from build123d import *

# Parameters (mm, degrees)
F0_W        = 102
F0_H        = 59.8
F0_W_2      = 98
F0_H_2      = 55.8
F1_DEPTH    = 8
F2_W        = 102.0620055497
F2_H        = 59.6651937813
F3_DEPTH    = 0.6
F4_W        = 100.1025550067
F4_H        = 57.5502440333
F4_W_2      = 98
F4_H_2      = 55.8
F5_DEPTH    = 2.5
F6_T1_DEPTH = 105.5349790349
F6_T3_DEPTH = 3.6684549434
F6_T5_DEPTH = 66.8066222098
F6_T7_DEPTH = 3.6684549117
F6_T9_DEPTH = 105.5349790665
F7_W        = 73
F7_H        = 27
F8_DEPTH    = 8.6010001


# Not quite as in the source:
# - a fillet or chamfer that OpenCascade refuses, or shapes differently, is made with other operations: its cross-section is extruded or revolved along the edge and cut away or added


with BuildPart() as f1:
    # F0 (on Top) → F1 (new body)
    with BuildSketch(Plane.XY):
        with Locations((-11.1629452705, -1.3489569187)):
            Rectangle(F0_W, F0_H)
        with Locations((-11.1629452705, -1.3489569187)):
            Rectangle(F0_W_2, F0_H_2, mode=Mode.SUBTRACT)
    extrude(amount=F1_DEPTH)

    # F2 (on Top) → F3 (join)
    with BuildSketch(Plane.XY):
        with Locations((-11.096207425, -1.3842275366)):
            Rectangle(F2_W, F2_H)
    extrude(amount=-F3_DEPTH)

    # F4 (on face) → F5 (join)
    with BuildSketch(Plane.XY.offset(8)):
        with Locations((-11.0803488642, -1.3563353568)):
            Rectangle(F4_W, F4_H)
        with Locations((-11.1629452705, -1.3489569187)):
            Rectangle(F4_W_2, F4_H_2, mode=Mode.SUBTRACT)
    extrude(amount=F5_DEPTH)

    # F6: fillet of radius 2 on 4 edges, made by hand

    # F6_s2 → F6_t1 (cut)
    with BuildSketch(Plane.YZ.offset(-65.6979244141)):
        with BuildLine():
            ThreePointArc((-29.7885387415, -0.6), (-30.5631354108, -0.4439088915), (-31.2168244272, 0))
            Line((-31.2168244272, 0), (-31.2168244272, -0.6))
            Line((-31.2168244272, -0.6), (-29.7885387415, -0.6))
        make_face()
    extrude(amount=F6_T1_DEPTH, mode=Mode.SUBTRACT)

    # F6_s4 → F6_t3 (cut)
    with BuildSketch(Plane.YZ.offset(39.8370546207)):
        with BuildLine():
            ThreePointArc((-29.7885387415, -0.6), (-30.5631354108, -0.4439088915), (-31.2168244272, 0))
            Line((-31.2168244272, 0), (-31.2168244272, -0.6))
            Line((-31.2168244272, -0.6), (-29.7885387415, -0.6))
        make_face()
    extrude(amount=F6_T3_DEPTH, mode=Mode.SUBTRACT)

    # F6_s6 → F6_t5 (cut)
    with BuildSketch(Plane.XZ.offset(-32.0190835683)):
        with BuildLine():
            ThreePointArc((-60.6989245141, -0.6), (-61.4735211834, -0.4439088915), (-62.1272101998, 0))
            Line((-62.1272101998, 0), (-62.1272101998, -0.6))
            Line((-62.1272101998, -0.6), (-60.6989245141, -0.6))
        make_face()
        with BuildLine():
            ThreePointArc((38.5065096641, -0.6), (39.2811063334, -0.4439088915), (39.9347953498, 0))
            Line((39.9347953498, 0), (39.9347953498, -0.6))
            Line((39.9347953498, -0.6), (38.5065096641, -0.6))
        make_face()
    extrude(amount=F6_T5_DEPTH, mode=Mode.SUBTRACT)

    # F6_s8 → F6_t7 (cut)
    with BuildSketch(Plane.YZ.offset(39.8370546524)):
        with BuildLine():
            ThreePointArc((28.448369354, 0), (27.7946803375, -0.4439088915), (27.0200836683, -0.6))
            Line((27.0200836683, -0.6), (28.448369354, -0.6))
            Line((28.448369354, -0.6), (28.448369354, 0))
        make_face()
    extrude(amount=F6_T7_DEPTH, mode=Mode.SUBTRACT)

    # F6_s10 → F6_t9 (cut)
    with BuildSketch(Plane.YZ.offset(-65.6979244141)):
        with BuildLine():
            ThreePointArc((28.448369354, 0), (27.7946803375, -0.4439088915), (27.0200836683, -0.6))
            Line((27.0200836683, -0.6), (28.448369354, -0.6))
            Line((28.448369354, -0.6), (28.448369354, 0))
        make_face()
    extrude(amount=F6_T9_DEPTH, mode=Mode.SUBTRACT)

    # F7 (on face) → F8 (cut, through all)
    with BuildSketch(Plane.XY.offset(8)):
        with Locations((-6.6629452705, 6.0510430813)):
            Rectangle(F7_W, F7_H)
    extrude(amount=-F8_DEPTH, mode=Mode.SUBTRACT)


solid = f1.part
The model under review builds one solid part; all positions refer to its coordinate system, in mm. A direction names the side the tool comes from. Round coordinates to 2 decimals unless told otherwise and drop trailing zeros. Loops run counter-clockwise (first coordinate to the right, second up) from the corner with the lowest first, then second, coordinate; pieces in that order, holes last. Notation, with made-up numbers: M 15.5,61.25 L 52.5,61.25 A18 cw 52.5,94.25 Z; hole C 13.25,-27.75 d3. An arc over 180 degrees is marked long. Answer as CSV lines item,"result". Start each with the question number.
Item 1: Mouldability with a two-part tool opening along X and no side actions: class faces 1 (the face through (38.971, -2, 9)), 2 (the face through (-12, -31.249, 4)), 3 (the face through (-12, -29.249, 5)) as released by +X, released by -X, zero draft, split by the parting line, or undercut.
Item 2: Insertion check: P1, Ø0.8, axis at x = -8, z = 10, coming from the +Y side; P2, Ø2, axis at y = 6.5, z = 8.5, coming from the +X side; P3, Ø1.2, axis at x = 3, z = 9.5, coming from the -Y side. Each pin has a flat end and moves straight along its axis. Give the tip position at first contact, or say it passes through.
Item 3: For faces 4 (the face through (-12, -13, 0)), 5 (the face through (39.837, -2, 4)), 6 (the face through (-12, -30.131, 9)), 7 (the face through (-61.132, -2, 9)), list the 3-axis set-ups (+Z, -Z, +X, -X, +Y, -Y) from which the entire face can be reached by the end or side of a thin tool; tool diameter is ignored.
Item 4: Wall thickness on line 1 (X direction, y = 8, z = 4); line 2 (Y direction, x = -1.5, z = 6.5); line 3 (X direction, y = -20, z = 9): over which ranges is each line inside the solid? List them lowest first. Write a range as [from, to].
Item 5: Consider section B-B (z = 7). Write out the cut boundary in (x, y).
Answer:
1,face 1,"released by +X"
1,face 2,"zero draft"
1,face 3,"undercut"
2,P1,"stops at y = 27.42"
2,P2,"stops at x = 39.84"
2,P3,"stops at y = -30.13"
3,face 4,"+Z"
3,face 5,"+Z, +X, +Y, -Y"
3,face 6,"+Z, +X, -X, -Y"
3,face 7,"+Z, -X, +Y, -Y"
4,line 1,"x = [-62.16, -60.16], [37.84, 39.84]"
4,line 2,"y = [-31.25, -29.25], [26.55, 28.55]"
4,line 3,"x = [-61.13, -60.16], [37.84, 38.97]"
5,outline,"M -62.16,-31.25 L 39.84,-31.25 L 39.84,28.55 L -62.16,28.55 Z; hole M -60.16,-29.25 L 37.84,-29.25 L 37.84,26.55 L -60.16,26.55 Z"
